Input: part model. Units: mm. Frame: model coordinates. Round coordinates to 2 decimals unless told otherwise and drop trailing zeros. Loops run counter-clockwise (first coordinate to the right, second up) from the corner with the lowest first, then second, coordinate; pieces in that order, holes last. Notation, with made-up numbers: (-7.5, 20.5) - (26.5, 20.5) arc R27 ccw to (26.5, 46.5) - close; hole circle Ø3 at (-11.75, 36.25). An arc over 180 degrees is marked (long way). One line per question, with ' | ' between items. Start each with the question number.
Item 1: Section B-B, the plane z = 0.5. Return loops of the section in (x, y).
Item 2: First-contact query: pin 1 (2 mm diameter, centred on y = 7.5, z = 4, fed in from +X); pin 2 (6 mm diameter, centred on x = -4, y = 11.5, fed in from -Z); pin 3 (1 mm diameter, centred on y = 10.5, z = 2.5, fed in from +X); pin 4 (2 mm diameter, centred on x = -11, z = 1, fed in from +Y). Flat tips, straight axial feed; report the tip coordinate or a pass-through.
Item 3: Section A-A, the plane z = 3.25. Return loops of the section in (x, y).
Item 4: Material intervals for line 1 along X through (y, z) = (1.5, 3); line 2 along Z through (x, y) = (2.5, -3.5); line 3 along Y through (x, z) = (3.5, 4.25), sorted ascending.
Item 5: Draft query along Y for faces 1 (the face through (0, 0, 1.5)), 2 (the face through (0, 0, 0)), 3 (the face through (11.17, 3.52, 5.79)). Return one class per face: pulls with the +Y half, pulls with the -Y half, needs draft (parallel to the pull), parting line crosses it, or undercut.
```python
from build123d import *

# Parameters (mm, degrees)
F0_R     = 17.5
F1_DEPTH = 10
F2_R     = 8
F3_DEPTH = 8.5
F5_R     = 2


# Not quite as in the source:
# - a fillet or chamfer that OpenCascade refuses, or shapes differently, is made with other operations: its cross-section is extruded or revolved along the edge and cut away or added


with BuildPart() as f1:
    # F0 (on Top) → F1 (new body)
    with BuildSketch(Plane.XY):
        Circle(F0_R)
    extrude(amount=F1_DEPTH)

    # F2 (on face) → F3 (cut)
    with BuildSketch(Plane.XY.offset(10)):
        Circle(F2_R)
    extrude(amount=-F3_DEPTH, mode=Mode.SUBTRACT)

    # F4: chamfer of 10 on 1 edges, made by hand

    # F4_s1 → F4_t2 (revolve, cut)
    with BuildSketch(Plane.XZ):
        Polygon((17.5, 0), (7.5, 10), (17.5, 10), align=None)
    revolve(axis=Axis((0, 0, 10), (0, 0, 1)), mode=Mode.SUBTRACT)

    # F5
    f5_edges = [f1.edges().sort_by_distance(p)[0] for p in [
        (-8, 0, 9.5),
    ]]
    fillet(f5_edges, radius=F5_R)


solid = f1.part
```
Return value:
1) outline: circle Ø34 at (0, 0)
2) pin 1: x = 12.55 | pin 2: z = 0 | pin 3: x = 11.54 | pin 4: y = 13.83
3) outline: circle Ø28.5 at (0, 0); hole circle Ø16 at (0, 0)
4) line 1: -14.42 to -7.86, 7.86 to 14.42 | line 2: 0 to 1.5 | line 3: -12.78 to -7.19, 7.19 to 12.78
5) face 1: undercut | face 2: needs draft | face 3: parting line crosses it
